Design review of the part built by this model. Coordinates are the model's own, in mm. Give positions to 0.01 mm unless a question says otherwise; leave off trailing zeros. Loops run counter-clockwise (first coordinate to the right, second up) from the corner with the lowest first, then second, coordinate; pieces in that order, holes last. Notation, with made-up numbers: (84, 65.5) - (125, 65.5) arc R8 cw to (125, 72.5) - close; hole circle Ø10 at (-32, 5.5). An arc over 180 degrees is marked (long way). Write each question's results on one line, items separated by ' | '.
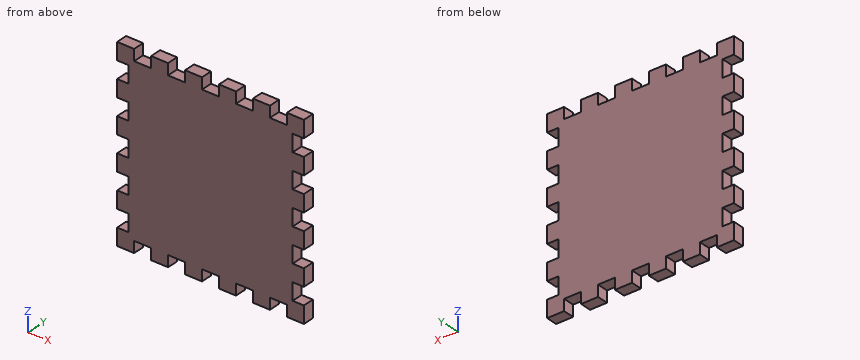
Autodesk Inventor part; units mm, degrees
ref_plane "YZ Plane" through (0, 0, 0) normal (1, 0, 0) x (0, 1, 0)
ref_plane "XZ Plane" through (0, 0, 0) normal (0, 1, 0) x (-1, 0, 0)
ref_plane "XY Plane" through (0, 0, 0) normal (0, 0, 1) x (1, 0, 0)
sketch "Sketch1" plane through (0, 0, 0) normal (0, 1, 0) x (-1, 0, 0)
  line L0 (20.4545, 25) -> (20.4545, 22)
  line L1 (15.9091, 22) -> (15.9091, 25)
  line L2 (11.3636, 25) -> (11.3636, 22)
  line L3 (6.8182, 22) -> (6.8182, 25)
  line L4 (2.2727, 25) -> (2.2727, 22)
  line L5 (-2.2727, 22) -> (-2.2727, 25)
  line L6 (-6.8182, 25) -> (-6.8182, 22)
  line L7 (-11.3636, 22) -> (-11.3636, 25)
  line L8 (-15.9091, 25) -> (-15.9091, 22)
  line L9 (-20.4545, 22) -> (-20.4545, 25)
  line L10 (-25, 20.4545) -> (-22, 20.4545)
  line L11 (-22, 15.9091) -> (-25, 15.9091)
  line L12 (-25, 11.3636) -> (-22, 11.3636)
  line L13 (-22, 6.8182) -> (-25, 6.8182)
  line L14 (-25, 2.2727) -> (-22, 2.2727)
  line L15 (-22, -2.2727) -> (-25, -2.2727)
  line L16 (-22, -6.8182) -> (-25, -6.8182)
  line L17 (-25, -11.3636) -> (-22, -11.3636)
  line L18 (-22, -15.9091) -> (-25, -15.9091)
  line L19 (-25, -20.4545) -> (-22, -20.4545)
  line L20 (-20.4545, -25) -> (-20.4545, -22)
  line L21 (-15.9091, -22) -> (-15.9091, -25)
  line L22 (-11.3636, -25) -> (-11.3636, -22)
  line L23 (-6.8182, -22) -> (-6.8182, -25)
  line L24 (-2.2727, -22) -> (-2.2727, -25)
  line L25 (2.2727, -25) -> (2.2727, -22)
  line L26 (20.4545, -22) -> (20.4545, -25)
  line L27 (15.9091, -25) -> (15.9091, -22)
  line L28 (11.3636, -22) -> (11.3636, -25)
  line L29 (6.8182, -25) -> (6.8182, -22)
  line L30 (22, -20.4545) -> (25, -20.4545)
  line L31 (25, -15.9091) -> (22, -15.9091)
  line L32 (25, -11.3636) -> (22, -11.3636)
  line L33 (25, -2.2727) -> (22, -2.2727)
  line L34 (25, 2.2727) -> (22, 2.2727)
  line L35 (25, 20.4545) -> (22, 20.4545)
  line L36 (22, 15.9091) -> (25, 15.9091)
  line L37 (25, 11.3636) -> (22, 11.3636)
  line L38 (22, 6.8182) -> (25, 6.8182)
  line L39 (15.9091, -22) -> (20.4545, -22)
  line L40 (6.8182, -22) -> (11.3636, -22)
  line L41 (-2.2727, -22) -> (2.2727, -22)
  line L42 (22, -20.4545) -> (22, -15.9091)
  line L43 (22, -2.2727) -> (22, 2.2727)
  line L44 (22, 6.8182) -> (22, 11.3636)
  line L45 (22, 15.9091) -> (22, 20.4545)
  line L46 (20.4545, 22) -> (15.9091, 22)
  line L47 (11.3636, 22) -> (6.8182, 22)
  line L48 (2.2727, 22) -> (-2.2727, 22)
  line L49 (-6.8182, 22) -> (-11.3636, 22)
  line L50 (-15.9091, 22) -> (-20.4545, 22)
  line L51 (-22, 20.4545) -> (-22, 15.9091)
  line L52 (-22, 11.3636) -> (-22, 6.8182)
  line L53 (-22, 2.2727) -> (-22, -2.2727)
  line L54 (-25, 6.8182) -> (-25, 2.2727)
  line L55 (-25, 25) -> (-25, 20.4545)
  line L56 (-25, 15.9091) -> (-25, 11.3636)
  line L57 (-20.4545, -22) -> (-15.9091, -22)
  line L58 (-11.3636, -22) -> (-6.8182, -22)
  line L59 (-22, -6.8182) -> (-22, -11.3636)
  line L60 (-22, -15.9091) -> (-22, -20.4545)
  line L61 (-25, -2.2727) -> (-25, -6.8182)
  line L62 (-25, -11.3636) -> (-25, -15.9091)
  line L63 (-25, -20.4545) -> (-25, -25)
  line L64 (-25, -25) -> (-20.4545, -25)
  line L65 (-15.9091, -25) -> (-11.3636, -25)
  line L66 (-6.8182, -25) -> (-2.2727, -25)
  line L67 (2.2727, -25) -> (6.8182, -25)
  line L68 (11.3636, -25) -> (15.9091, -25)
  line L69 (20.4545, -25) -> (25, -25)
  line L70 (25, -25) -> (25, -20.4545)
  line L71 (25, 2.2727) -> (25, 6.8182)
  line L72 (25, 11.3636) -> (25, 15.9091)
  line L73 (25, 20.4545) -> (25, 25)
  line L74 (25, 25) -> (20.4545, 25)
  line L75 (15.9091, 25) -> (11.3636, 25)
  line L76 (6.8182, 25) -> (2.2727, 25)
  line L77 (-2.2727, 25) -> (-6.8182, 25)
  line L78 (-11.3636, 25) -> (-15.9091, 25)
  line L79 (-20.4545, 25) -> (-25, 25)
  line L80 (22, -11.3636) -> (22, -6.8182)
  line L81 (22, -6.8182) -> (25, -6.8182)
  line L82 (25, -15.9091) -> (25, -11.3636)
  line L83 (25, -6.8182) -> (25, -2.2727)
  point P0 (0, 0)
  dimension "d1" = 50
  dimension "d3" = 50
  dimension "d5" = 25
  dimension "d6" = 25
  dimension "d7" = 3
  dimension "d8" = 3
  dimension "d9" = 3
  dimension "d10" = 3
  dimension "d15" = 4.5454
extrude "Extrusion1" add sketch "Sketch1" along normal blind 3
equation "\"d1\" = wt"
equation "\"d3\" = lt"
equation "\"d7\" = tt"
equation "\"d8\" = tt"
equation "\"d9\" = tt"
equation "\"d10\" = tt"
equation "\"d13\" = tt"
equation "\"wt\" = 50"
equation "\"tt\" = 3"
equation "\"tol\" = 0"
equation "\"tiroir\" = 25.4"
equation "\"nHoles\" = 101.6"
equation "\"shelfH\" = 35"
equation "\"d0\" = 0.5 * wt"
equation "\"d2\" = 0.5 * lt"
equation "\"lt\" = 50"
equation "\"d4\" = tt"
properties part number "base"
Item 1: Wall thickness on probe 1 along Z at (x, y) = (-23, 0.2); probe 2 along X at (y, z) = (2.05, -19.5): over which ranges is each line inside the solid? List them lowest first.
Output values:
probe 1: z = -25 to -20.45, -15.91 to -11.36, -6.82 to -2.27, 2.27 to 6.82, 11.36 to 15.91, 20.45 to 25 | probe 2: x = -22 to 22
Item 2: We need section B-B on z = -16.5. Give the boundary of the cut face in (x, y).
Output values:
outline: (-22, 0) - (22, 0) - (22, 3) - (-22, 3) - close
Item 3: We need section A-A on x = 17.5. Give the boundary of the cut face in (y, z), then the cut area to 3 significant figures.
Output values:
outline: (0, -22) - (3, -22) - (3, 22) - (0, 22) - close | area: 132 mm²
Item 4: Clearance check with flat-ended pins moving along their axes: P1, Ø0.9, axis at x = -8.5, y = 1, coming from the +Z side; P2, Ø1.5, axis at y = 1, z = 18.5, coming from the +X side. State where each tip first meets the part, or that it passes through.
Output values:
P1: stops at z = 22 | P2: stops at x = 22
